Here's how the part is built. I have some questions about the finished solid (model axes, mm). A direction names the side the tool comes from. Round coordinates to 2 decimals unless told otherwise and drop trailing zeros. Write each loop counter-clockwise with the first axis right and the second up, starting at its lowest first coordinate (ties: lowest second). Pieces come first, ordered by that corner, then holes. Notation, with made-up numbers: (-40, -37) -> (3, -37) arc R8 ccw to (3, -29) -> close; hole circle Ø1 at (34, -4). An arc over 180 degrees is marked (long way). Answer in a Markdown table with one row per item.
from build123d import *

# Parameters (mm, degrees)
SKETCH1_W           = 762
SKETCH1_H           = 762
SKETCH1_W_2         = 25.4
SKETCH1_H_2         = 635
BOSS_EXTRUDE1_DEPTH = 3
SKETCH2_W           = 50.8
SKETCH2_H           = 762
BOSS_EXTRUDE2_DEPTH = 76.2


with BuildPart() as part:
    # Sketch1 → Boss-Extrude1 (new, symmetric)
    with BuildSketch(Plane(origin=(0, 0, 0), x_dir=(1, 0, 0), z_dir=(0, 1, 0))):
        Rectangle(SKETCH1_W, SKETCH1_H)
        with Locations((-249.2248, 0)):
            Rectangle(SKETCH1_W_2, SKETCH1_H_2, mode=Mode.SUBTRACT)
        with Locations((249.2248, 0)):
            Rectangle(SKETCH1_W_2, SKETCH1_H_2, mode=Mode.SUBTRACT)
    extrude(amount=BOSS_EXTRUDE1_DEPTH, both=True)

    # Sketch2 → Boss-Extrude2 (add)
    with BuildSketch(Plane(origin=(0, 3, 0), x_dir=(1, 0, 0), z_dir=(0, 1, 0))):
        Rectangle(SKETCH2_W, SKETCH2_H)
    extrude(amount=BOSS_EXTRUDE2_DEPTH)


solid = part.part
1) I want a section at C-C, the plane y = 23.5. List the corners of the cut face in (x, z) for me, and give its area (3 significant figures).
Response:
| item | result |
|---|---|
| outline | (-25.4, -381) -> (25.4, -381) -> (25.4, 381) -> (-25.4, 381) -> close |
| area | 38,700 mm^2 |
2) I need wall thicknesses on line 1 (X direction, y = 31.5, z = -32); line 2 (Y direction, x = -335, z = 139). Which ranges of each line are inside material? Lowest first, please. Write a range as [from, to].
Response:
| item | result |
|---|---|
| line 1 | x = [-25.4, 25.4] |
| line 2 | y = [-3, 3] |
3) I want a section at D-D, the plane x = 204. List the corners of the cut face in (y, z) for me, and give its area (3 significant figures).
Response:
| item | result |
|---|---|
| outline | (-3, -381) -> (3, -381) -> (3, 381) -> (-3, 381) -> close |
| area | 4,570 mm^2 |
4) Which directions (+Z, -Z, +X, -X, +Y, -Y) give clear straight access to the entire face, cutting with the end or side of a thin tool? Please do faces 1 (the face through (-25.4, 41, 5)), 2 (the face through (201, 3, -5)), 3 (the face through (-2, 14, 381)).
Response:
| item | result |
|---|---|
| face 1 | +Z, -Z, -X, +Y |
| face 2 | +Z, -Z, +X, +Y |
| face 3 | +Z, +X, -X, +Y, -Y |
5) I want a section at B-B, the plane z = -329. List the corners of the cut face in (x, y) for me, and give its area (3 significant figures).
Response:
| item | result |
|---|---|
| outline | (-381, -3) -> (381, -3) -> (381, 3) -> (25.4, 3) -> (25.4, 79.2) -> (-25.4, 79.2) -> (-25.4, 3) -> (-381, 3) -> close |
| area | 8,440 mm^2 |
6) I want a section at A-A, the plane z = 3. List the corners of the cut face in (x, y) for me, and give its area (3 significant figures).
Response:
| item | result |
|---|---|
| outline | (-381, -3) -> (-261.92, -3) -> (-261.92, 3) -> (-381, 3) -> close; (-236.52, -3) -> (236.52, -3) -> (236.52, 3) -> (25.4, 3) -> (25.4, 79.2) -> (-25.4, 79.2) -> (-25.4, 3) -> (-236.52, 3) -> close; (261.92, -3) -> (381, -3) -> (381, 3) -> (261.92, 3) -> close |
| area | 8,140 mm^2 |
7) For pin 1 (10 mm diameter, centred on y = 56.5, z = -167.5, fed in from +X); pin 2 (1 mm diameter, centred on x = 148, z = -158, fed in from +Y), each with a flat end and sliding along its axis, tell me the tip position at first contact or that it passes through.
Response:
| item | result |
|---|---|
| pin 1 | stops at x = 25.4 |
| pin 2 | stops at y = 3 |
